```python
from build123d import *

# Parameters (mm, degrees)
SKETCH1_W           = 310
SKETCH1_H           = 280
SKETCH1_W_2         = 285
SKETCH1_H_2         = 255
BOSS_EXTRUDE1_DEPTH = 43
SKETCH2_R           = 1.5
CUT_EXTRUDE1_DEPTH  = 10


with BuildPart() as part:
    # Sketch1 → Boss-Extrude1 (new body)
    with BuildSketch(Plane(origin=(0, 0, 0), x_dir=(1, 0, 0), z_dir=(0, 1, 0))):
        with Locations((155, 140)):
            Rectangle(SKETCH1_W, SKETCH1_H)
        with Locations((155, 140)):
            Rectangle(SKETCH1_W_2, SKETCH1_H_2, mode=Mode.SUBTRACT)
    extrude(amount=BOSS_EXTRUDE1_DEPTH)

    # Sketch2 → Cut-Extrude1 (cut)
    with BuildSketch(Plane(origin=(0, 43, 0), x_dir=(1, 0, 0), z_dir=(0, 1, 0))):
        with Locations(Location((303.75, 243.75, 0), (0, 0, 270))):
            Circle(SKETCH2_R)
        with Locations(Location((303.75, 223.75, 0), (0, 0, 270))):
            Circle(SKETCH2_R)
        with Locations(Location((303.75, 56.25, 0), (0, 0, 270))):
            Circle(SKETCH2_R)
        with Locations(Location((303.75, 36.25, 0), (0, 0, 270))):
            Circle(SKETCH2_R)
    extrude(amount=-CUT_EXTRUDE1_DEPTH, mode=Mode.SUBTRACT)


solid = part.part
```
Part model, mm, in its own coordinate system. A direction names the side the tool comes from. Round coordinates to 2 decimals unless told otherwise and drop trailing zeros. Loops run counter-clockwise (first coordinate to the right, second up) from the corner with the lowest first, then second, coordinate; pieces in that order, holes last. Notation, with made-up numbers: (-28, -10) -> (-8, -10) arc R24 ccw to (-8, 24) -> close; hole circle Ø10 at (71, 25.5). An arc over 180 degrees is marked (long way). Use one line per item in the form item = value. Start each with the question number.
Item 1: Two-plate mould, pull along Z, no slides. Class faces 1 (the flat face through (153, 21, -12.5)), 2 (the flat face through (153, 21, 0)), 3 (the flat face through (143, 43, -275)): released by +Z, released by -Z, zero draft, split by the parting line, or undercut.
Item 2: Tool access for faces 4 (the flat face through (310, 21, -138)), 5 (the flat face through (12.5, 21, -138)): list every direction of +Z, -Z, +X, -X, +Y, -Y with a clear straight run to the whole face (end or side of a thin tool).
Item 3: Band-saw the part on C-C (y = 11). List the corners of the cut face in (x, z), plus the area to 3 significant figures.
Item 4: Band-saw the part on B-B (z = -162). List the corners of the cut face in (x, y).
Item 5: Band-saw the part on A-A (x = 268). List the corners of the cut face in (y, z).
Item 6: Drill centre lines: line 1 along X through (y, z) = (35.25, -36.25); line 2 along Z through (x, y) = (303.75, 39); line 3 along Z through (x, y) = (117.5, 9). Where is each one in solid material? Low to high.
Item 7: Drop flat-ended pins along their axis: pin 1 Ø4 at (x, y) = (136.5, 20.5) entering from +Z; pin 2 Ø1.5 at (x, z) = (303.5, -36.5) entering from +Y. Give the stop position or say it passes through.
Data:
q1.face_1 = undercut
q1.face_2 = released by +Z
q1.face_3 = zero draft
q2.face_4 = +Z, -Z, +X, +Y, -Y
q2.face_5 = +Y, -Y
q3.outline = (0, -280) -> (310, -280) -> (310, 0) -> (0, 0) -> close; hole (12.5, -267.5) -> (297.5, -267.5) -> (297.5, -12.5) -> (12.5, -12.5) -> close
q3.area = 14,100 mm^2
q4.outline = (0, 0) -> (12.5, 0) -> (12.5, 43) -> (0, 43) -> close; (297.5, 0) -> (310, 0) -> (310, 43) -> (297.5, 43) -> close
q5.outline = (0, -280) -> (43, -280) -> (43, -267.5) -> (0, -267.5) -> close; (0, -12.5) -> (43, -12.5) -> (43, 0) -> (0, 0) -> close
q6.line_1 = 0 to 12.5, 297.5 to 302.25, 305.25 to 310
q6.line_2 = -280 to -245.25, -242.25 to -225.25, -222.25 to -57.75, -54.75 to -37.75, -34.75 to 0
q6.line_3 = -280 to -267.5, -12.5 to 0
q7.pin_1 = 0
q7.pin_2 = 33
